Can you work these out from the model? Positions are in its coordinate system, mm. Face numbers are marked on the shaded views. Round coordinates to 2 decimals unless told otherwise and drop trailing zeros. Write each loop counter-clockwise with the first axis right and the second up, starting at its lowest first coordinate (ties: lowest second). Pieces come first, ordered by that corner, then holes. Notation, with made-up numbers: (-9, 73.5) - (2, 73.5) arc R34 cw to (2, 111.5) - close; hole circle Ø1 at (15.5, 71). An arc over 180 degrees is marked (long way). One line per item, written item: value. Start each with the question number.
(1) If I drill on L1, parallel to X at y = 116.5, z = -13; L2, parallel to Y at x = 22, z = 0.5; L3, parallel to Y at x = 145.5, z = 1.5, over which ranges is the centre line in solid material (lowest first)? Write a range as from..to.
(2) I want a section at D-D on x = 122. List the corners of the cut face in (y, z) for me, plus the area to 3 significant figures.
(3) I'm going to push flat-ended pins straight in: pin 1 Ø1.8 at (y, z) = (45.85, -8) entering from +X; pin 2 Ø1.5 at (x, y) = (140.5, 74.5) entering from +Z; pin 3 Ø5 at (x, z) = (132, 3) entering from -Y; pin 4 Ø5 at (x, z) = (21.5, 6) entering from +Y. Where does each tip first touch, or does it pass through?
(4) I want a section at B-B on z = 12.5. List the corners of the cut face in (x, y) for me.
(5) I want a section at A-A on y = -14. List the corners of the cut face in (x, z) for me (3 decimals), plus the area to 3 significant figures.
(6) I want a section at C-C on y = 53.5. List the corners of the cut face in (x, z) for me (3 decimals).
(7) Thinking about a two-plate mould opening in X: for the marked faces 1, 2, 3 and 4, which applies, +X half, -X half, draft (parallel to the pull), parting line (faces both ways), or undercut?
from build123d import *

# Parameters (mm, degrees)
SKETCH_1_W          = 220
SKETCH_1_H          = 120
EXTRUDE_1_DEPTH     = 10
CUT_EXTRUDE_1_DEPTH = 10
SKETCH_5_R          = 1
SKETCH_5_W          = 10
SKETCH_5_H          = 110
EXTRUDE_2_DEPTH     = 5


with BuildPart() as part:
    # 草图1 → 凸台-拉伸1 (new body)
    with BuildSketch(Plane.XY):
        with Locations((110, 60)):
            Rectangle(SKETCH_1_W, SKETCH_1_H)
    extrude(amount=EXTRUDE_1_DEPTH)

    # 草图2 → 切除-拉伸1 (cut)
    with BuildSketch(Plane.XY.offset(10)):
        Polygon((220, 120), (30, 120), (30, 80), (190, 80), (190, 115), (220, 115), align=None)
        Polygon((220, 0), (220, 5), (190, 5), (190, 40), (30, 40), (30, 0), align=None)
    extrude(amount=-CUT_EXTRUDE_1_DEPTH, mode=Mode.SUBTRACT)

    # 草图5 → 凸台-拉伸2 (add)
    # profile 1 of 3: a face of its own
    with BuildSketch(Plane(origin=(220, 0, 0), x_dir=(0, 0, -1), z_dir=(1, 0, 0))):
        with BuildLine():
            Line((-27.365, 70.42619968), (-27.365, 159.57380032))
            ThreePointArc((-27.365, 159.57380032), (-5, 164.87), (17.365, 159.57380032))
            Line((17.365, 159.57380032), (17.365, 70.42619968))
            Line((17.365, 70.42619968), (17.365, 49.57380032))
            Line((17.365, 49.57380032), (17.365, -39.57380032))
            ThreePointArc((17.365, -39.57380032), (-5, -44.87), (-27.365, -39.57380032))
            Line((-27.365, -39.57380032), (-27.365, 49.57380032))
            Line((-27.365, 49.57380032), (-27.365, 70.42619968))
        make_face()
        with Locations((-5, 157.87)):
            Circle(SKETCH_5_R, mode=Mode.SUBTRACT)
        with Locations((-18, 155.851400221)):
            Circle(SKETCH_5_R, mode=Mode.SUBTRACT)
        with Locations((8, 155.851400221)):
            Circle(SKETCH_5_R, mode=Mode.SUBTRACT)
        with Locations((8, 74.148599779)):
            Circle(SKETCH_5_R, mode=Mode.SUBTRACT)
        with Locations((-18, 74.148599779)):
            Circle(SKETCH_5_R, mode=Mode.SUBTRACT)
        with Locations((-18, 45.851400221)):
            Circle(SKETCH_5_R, mode=Mode.SUBTRACT)
        with Locations((8, 45.851400221)):
            Circle(SKETCH_5_R, mode=Mode.SUBTRACT)
        with Locations((8, -35.851400221)):
            Circle(SKETCH_5_R, mode=Mode.SUBTRACT)
        with Locations((-18, -35.851400221)):
            Circle(SKETCH_5_R, mode=Mode.SUBTRACT)
        with Locations((-5, -37.87)):
            Circle(SKETCH_5_R, mode=Mode.SUBTRACT)
        with Locations((-5, 60)):
            Rectangle(SKETCH_5_W, SKETCH_5_H, mode=Mode.SUBTRACT)
    # profile 2 of 3: a face of its own
    with BuildSketch(Plane(origin=(220, 0, 0), x_dir=(0, 0, -1), z_dir=(1, 0, 0))):
        with Locations((-5, 47.87)):
            Circle(SKETCH_5_R)
    # profile 3 of 3: a face of its own
    with BuildSketch(Plane(origin=(220, 0, 0), x_dir=(0, 0, -1), z_dir=(1, 0, 0))):
        with Locations((-5, 72.13)):
            Circle(SKETCH_5_R)
    extrude_2 = extrude(amount=-EXTRUDE_2_DEPTH)

    # 镜向1: 凸台-拉伸2 across plane
    add(extrude_2.mirror(Plane(origin=(110, 0, 0), x_dir=(0, 0, 1), z_dir=(1, 0, 0))))


solid = part.part
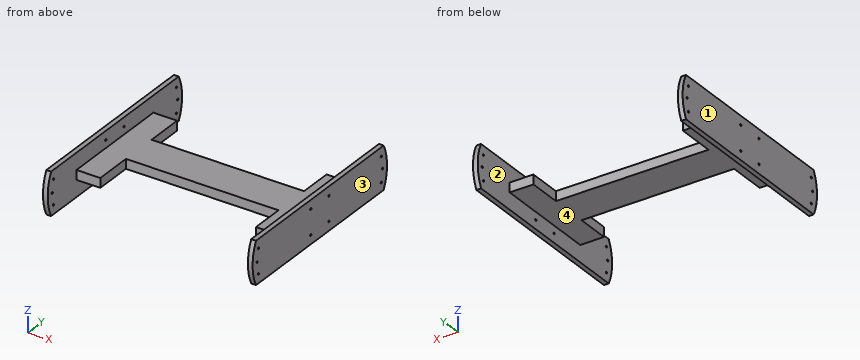
Established:
1. L1: 0..5, 215..220
1. L2: 0..120
1. L3: 40..80
2. outline: (40, 0) - (80, 0) - (80, 10) - (40, 10) - close
2. area: 400 mm2
3. pin 1: through
3. pin 2: z = 10
3. pin 3: y = 40
3. pin 4: y = 120
4. outline: (0, -44.3) - (5, -44.3) - (5, 164.3) - (0, 164.3) - close; (215, -44.3) - (220, -44.3) - (220, 164.3) - (215, 164.3) - close
5. outline: (0, -17.365) - (5, -17.365) - (5, 27.365) - (0, 27.365) - close; (215, -17.365) - (220, -17.365) - (220, 27.365) - (215, 27.365) - close
5. area: 447 mm2
6. outline: (0, -17.365) - (5, -17.365) - (5, 0) - (215, 0) - (215, -17.365) - (220, -17.365) - (220, 27.365) - (215, 27.365) - (215, 10) - (5, 10) - (5, 27.365) - (0, 27.365) - close
7. face 1: -X half
7. face 2: undercut
7. face 3: +X half
7. face 4: undercut
